Source: CAD feature listing. Evaluate the final solid. Frame: model axes, mm. A direction names the side the tool comes from. Give positions to 0.01 mm unless a question says otherwise; leave off trailing zeros. Write each loop counter-clockwise with the first axis right and the second up, starting at its lowest first coordinate (ties: lowest second). Pieces come first, ordered by that corner, then holes. Notation, with made-up numbers: M 35.25,74 L 63.25,74 A20 ccw 63.25,109 Z; hole C -23,1.25 d6. An arc over 180 degrees is marked long. Use CSV: the item, a comma, the result in double quotes. Start each with the question number.
from build123d import *

# Parameters (mm, degrees)
F0_R     = 30
F1_DEPTH = 3
F2_R     = 9
F3_DEPTH = 50
F4_T     = 1.5


# Not quite as in the source:
# - a shell that OpenCascade refuses in one call is made with other operations: the cavity is built on its own and cut out


with BuildPart() as f1:
    # F0 (on Top) → F1 (new body)
    with BuildSketch(Plane.XY):
        Circle(F0_R)
    extrude(amount=F1_DEPTH)

    # F2 (on face) → F3 (join)
    with BuildSketch(Plane.XY.offset(3)):
        Circle(F2_R)
    extrude(amount=F3_DEPTH)

    # F4: shell of thickness 1.5, made by hand


with BuildPart() as f4_core1:
    # F4_t2: copy of F1
    add(f1.part)

    # the walls: a layer under each face that stays
    f4_faces = [f4_core1.faces().sort_by_distance(p)[0] for p in [
        (-30, 0, 1.5),
        (0, 0, 0),
        (-20, -20, 3),
        (-9, 0, 28),
    ]]
    thicken(f4_faces, amount=-F4_T, mode=Mode.SUBTRACT)

    # F4_s3 → F4_t4 (revolve, cut)
    with BuildSketch(Plane.XZ):
        Polygon((9.015, 3.015), (9, 1.5), (7.5, 1.5), (7.5, 3), align=None)
    revolve(axis=Axis((0, 0, 3), (0, 0, 1)), mode=Mode.SUBTRACT)


with BuildPart() as f1_1:
    add(f1.part)

    # what is left inside the walls is the cavity
    f4_cavity = [f4_core1.part.solids().sort_by_distance(p)[0] for p in [
        (-7.485, 0, 18.666667),
    ]]
    add(f4_cavity, mode=Mode.SUBTRACT)


solid = f1_1.part
1. Section C-C on z = 15.5. Return loops of the section in (x, y).
2. Pull-direction query (Y, two-part tool) for faces 1 (the cylindrical face through (-7.493, 0.33, 27.61)), 2 (the cylindrical face through (-1.172, 8.923, 27.65)), 3 (the flat face through (6, 7, 3)); classes: released by +Y, released by -Y, zero draft, split by the parting line, or undercut.
3. First-contact query: pin 1 (1.5 mm diameter, centred on x = 5.5, z = 23, fed in from -Y); pin 2 (13.5 mm diameter, centred on x = 0, y = 0, fed in from +Z); pin 3 (1.5 mm diameter, centred on y = 4.5, z = 31, fed in from +X). Flat tips, straight axial feed; report the tip coordinate or a pass-through.
4. Access query for faces 4 (the cylindrical face through (-29.97, 1.32, 1.48)), 5 (the flat face through (0, 0, 1.5)). Directions: +Z, -Z, +X, -X, +Y, -Y. A direction counts if a zero-diameter tool reaches every point of the face in a straight line with its end or side. Return the directions, or none.
5. Section A-A on y = 0. Return loops of the section in (x, z), then the cut area to 4 significant figures.
6. Section D-D on y = -24. Return loops of the section in (x, z).
7. Line query: probe 1 along Y at (x, z) = (0, 16); probe 2 along Z at (x, y) = (-10.5, -13); probe 3 along X at (y, z) = (2, 16). Output: solid intervals per line, ascending.
Resolved:
1,outline,"C 0,0 d18; hole C 0,0 d15"
2,face 1,"undercut"
2,face 2,"split by the parting line"
2,face 3,"zero draft"
3,pin 1,"stops at y = -7.64"
3,pin 2,"stops at z = 1.5"
3,pin 3,"stops at x = 8.18"
4,face 4,"+Z, -Z"
4,face 5,"+Z"
5,outline,"M -30,0 L 30,0 L 30,3 L 9,3 L 9,53 L 7.5,53 L 7.5,1.5 L -7.5,1.5 L -7.5,53 L -9,53 L -9,3 L -30,3 Z"
5,area,"307.5 mm2"
6,outline,"M -18,0 L 18,0 L 18,3 L -18,3 Z"
7,probe 1,"y = -9 to -7.5, 7.5 to 9"
7,probe 2,"z = 0 to 3"
7,probe 3,"x = -8.77 to -7.23, 7.23 to 8.77"
